from build123d import *

# Parameters (mm, degrees)
SALIENTE_EXTRUIR1_DEPTH = 5


with BuildPart() as part:
    # Croquis1 → Saliente-Extruir1 (new body)
    with BuildSketch(Plane(origin=(0, 0, 0), x_dir=(0, 0, -1), z_dir=(1, 0, 0))):
        Polygon((-17.15051747, 72.789115646), (-17.15051747, 62.789115646), (-12.15051747, 62.789115646), (-12.15051747, 52.789115646), (-17.15051747, 52.789115646), (-17.15051747, 42.789115646), (-12.15051747, 42.789115646), (-12.15051747, 32.789115646), (-17.15051747, 32.789115646), (-17.15051747, 22.789115646), (-12.15051747, 22.789115646), (-12.15051747, 12.789115646), (-17.15051747, 12.789115646), (-17.15051747, 2.789115646), (-12.15051747, 2.789115646), (-12.15051747, -7.210884354), (-17.15051747, -7.210884354), (-17.15051747, -17.210884354), (-12.15051747, -17.210884354), (-12.15051747, -27.210884354), (-17.15051747, -27.210884354), (-17.15051747, -37.210884354), (-12.15051747, -37.210884354), (-12.15051747, -47.210884354), (-17.15051747, -47.210884354), (-17.15051747, -57.210884354), (-12.15051747, -57.210884354), (-12.15051747, -67.210884354), (-5.15051747, -67.210884354), (-5.15051747, -57.210884354), (-0.15051747, -57.210884354), (-0.15051747, -47.210884354), (-5.15051747, -47.210884354), (-5.15051747, -37.210884354), (-0.15051747, -37.210884354), (-0.15051747, -27.210884354), (-5.15051747, -27.210884354), (-5.15051747, -17.210884354), (-0.15051747, -17.210884354), (-0.15051747, -7.210884354), (-5.15051747, -7.210884354), (-5.15051747, 2.789115646), (-0.15051747, 2.789115646), (-0.15051747, 12.789115646), (-5.15051747, 12.789115646), (-5.15051747, 22.789115646), (-0.15051747, 22.789115646), (-0.15051747, 32.789115646), (-5.15051747, 32.789115646), (-5.15051747, 42.789115646), (-0.15051747, 42.789115646), (-0.15051747, 52.789115646), (-5.15051747, 52.789115646), (-5.15051747, 62.789115646), (-0.15051747, 62.789115646), (-0.15051747, 72.789115646), (-5.15051747, 72.789115646), (-5.15051747, 82.789115646), (-0.15051747, 82.789115646), (-0.15051747, 92.789115646), (-17.15051747, 92.789115646), (-17.15051747, 82.789115646), (-12.15051747, 82.789115646), (-12.15051747, 72.789115646), align=None)
    extrude(amount=SALIENTE_EXTRUIR1_DEPTH)


solid = part.part
CAD build for the part. Positions are in the model's coordinates, mm. A direction names the side the tool comes from. Round coordinates to 2 decimals unless told otherwise and drop trailing zeros. Write each loop counter-clockwise with the first axis right and the second up, starting at its lowest first coordinate (ties: lowest second). Pieces come first, ordered by that corner, then holes.
(1) Drop flat-ended pins along their axis: P1, Ø1.5, axis at x = 1.5, y = 20, coming from the +Z side; P2, Ø1.5, axis at x = 3.5, y = -63, coming from the -Z side; P3, Ø3, axis at x = 1.5, z = 3.5, coming from the -Y side. Give the stop position or say it passes through.
(2) Probe line 1 along Z through (x, y) = (0.8, -38.5). List the from-to ranges inside material, lowest first.
(3) Slice it at B-B, the plane y = -45. Write the cut outline in (x, z).
(4) Mould opens along Y. For faces 4 (the face through (5, 32, 9)), 5 (the face through (2, 92.789, 9)), 6 (the face through (2, -2, 5.151)), 7 (the face through (2, 2.789, 15)) say: pulls with the +Y half, pulls with the -Y half, needs draft (parallel to the pull), parting line crosses it, or undercut.
(5) 3-axis set-ups, long thin cutter, end or side, ignore diameter. For faces 1 (the face through (2, 38, 12.151)), 2 (the face through (2, 48, 0.151)), 3 (the face through (2, 42.789, 3)): which of +Z, -Z, +X, -X, +Y, -Y reach the whole face in a straight line?
(6) Slice it at A-A, the plane z = 1.5. Count the separate pieces of the cut face and the enclosed holes in it, and give its area (3 significant figures).
From the geometry:
1. P1: stops at z = 12.15
1. P2: stops at z = 5.15
1. P3: stops at y = -57.21
2. line 1: z = 5.15 to 12.15
3. outline: (0, 5.15) - (5, 5.15) - (5, 12.15) - (0, 12.15) - close
4. face 4: needs draft
4. face 5: pulls with the +Y half
4. face 6: undercut
4. face 7: undercut
5. face 1: +Z, +X, -X
5. face 2: -Z, +X, -X, +Y, -Y
5. face 3: -Z, +X, -X
6. separate pieces: 8
6. enclosed holes: 0
6. area: 400 mm2
